Here's how the part is built. I have some questions about the finished solid (model axes, mm). A direction names the side the tool comes from. Coordinates: 2 decimals unless noted, no trailing zeros. Order: outer loops, then holes, each group sorted by start corner. A loop starts at its lowest first (then second) coordinate and runs counter-clockwise, first axis right, second up. Notation, with made-up numbers: M 6,55 L 24,55 A32 ccw 24,87 Z; hole C -40,35 d2. An arc over 180 degrees is marked long. Answer as CSV lines item,"result". Start each with the question number.
```python
from build123d import *

# Parameters (mm, degrees)
SKETCH1_R           = 15
BOSS_EXTRUDE1_DEPTH = 5
SKETCH2_R           = 5
BOSS_EXTRUDE2_DEPTH = 90
CUT_EXTRUDE1_START  = -15
CUT_EXTRUDE1_DEPTH  = 15
SKETCH4_W           = 2
SKETCH4_H           = 5.2
CUT_EXTRUDE2_DEPTH  = 99.17076958
FILLET1_R           = 10
FILLET2_R           = 2
CUT_EXTRUDE3_DEPTH  = 1
SKETCH6_R           = 13.5
SKETCH6_R_2         = 11.5
CUT_EXTRUDE4_DEPTH  = 1


with BuildPart() as part:
    # Sketch1 → Boss-Extrude1 (new body)
    with BuildSketch(Plane(origin=(0, 0, 0), x_dir=(1, 0, 0), z_dir=(0, 1, 0))):
        with Locations(Location((0, 0, 0), (0, 0, 270))):
            Circle(SKETCH1_R)
    extrude(amount=BOSS_EXTRUDE1_DEPTH)

    # Sketch2 → Boss-Extrude2 (add)
    with BuildSketch(Plane(origin=(0, 5, 0), x_dir=(1, 0, 0), z_dir=(0, 1, 0))):
        with Locations(Location((0, 0, 0), (0, 0, 90))):
            Circle(SKETCH2_R)
    extrude(amount=BOSS_EXTRUDE2_DEPTH)

    # Sketch3 → Cut-Extrude1 (cut)
    with BuildSketch(Plane(origin=(0, 95, 0), x_dir=(1, 0, 0), z_dir=(0, 1, 0)).offset(CUT_EXTRUDE1_START)):
        with BuildLine():
            Line((0, 5), (5, 0))
            ThreePointArc((5, 0), (3.535533906, 3.535533906), (0, 5))
        make_face()
    extrude(amount=CUT_EXTRUDE1_DEPTH, mode=Mode.SUBTRACT)

    # Sketch4 → Cut-Extrude2 (cut, through all)
    with BuildSketch(Plane(origin=(2.5, 0, -2.5), x_dir=(-0.7071067811865475, 0, -0.7071067811865477), z_dir=(0.7071067811865477, 0, -0.7071067811865475))):
        with Locations((0, 87.5)):
            Rectangle(SKETCH4_W, SKETCH4_H)
    extrude(amount=-CUT_EXTRUDE2_DEPTH, mode=Mode.SUBTRACT)

    # Fillet1
    fillet1_edges = [part.edges().sort_by_distance(p)[0] for p in [
        (0, 5, 5),
    ]]
    fillet(fillet1_edges, radius=FILLET1_R - 0.0001)  # a hair under: the kernel refuses the full size

    # Fillet2
    fillet2_edges = [part.edges().sort_by_distance(p)[0] for p in [
        (0, 5, -15),
    ]]
    fillet(fillet2_edges, radius=FILLET2_R)

    # Sketch5 → Cut-Extrude3 (cut)
    with BuildSketch(Plane.XZ):
        with BuildLine():
            Line((-0.690387564, 10.623320935), (9.77235282, 0.16058055))
            Line((9.77235282, 0.16058055), (7.687016282, -1.924755988))
            Line((7.687016282, -1.924755988), (-2.195796218, 3.006133435))
            add(Edge.make_bspline(
                [(-2.195796218, 3.006133435), (-2.307029511, 3.062113904), (-2.52269645, 3.170652781), (-2.833890677, 3.329506222), (-3.122930247, 3.477577181), (-3.391022331, 3.612480856), (-3.636978399, 3.737620248), (-3.85910859, 3.856159494), (-4.059958905, 3.960316417), (-4.186011343, 4.026707574), (-4.245075064, 4.057816127)],
                knots=[0, 0, 0, 0, 1.297460102, 2.515607, 3.640415016, 4.681187102, 5.642653462, 6.515599393, 7.304462283, 8, 8, 8, 8], degree=3))
            add(Edge.make_bspline(
                [(-4.245075064, 4.057816127), (-4.210973718, 3.991734504), (-4.138662994, 3.851610709), (-4.025441526, 3.629760807), (-3.897989309, 3.38652834), (-3.762956902, 3.118983989), (-3.620144132, 2.827316511), (-3.462218864, 2.515142559), (-3.297896109, 2.177641474), (-3.18347293, 1.945388515), (-3.124281795, 1.825244012)],
                knots=[0, 0, 0, 0, 0.714390188, 1.514839662, 2.392796159, 3.352429004, 4.393822708, 5.512665897, 6.71330155, 8, 8, 8, 8], degree=3))
            Line((-3.124281795, 1.825244012), (1.650357628, -7.961414642))
            Line((1.650357628, -7.961414642), (-0.212623141, -9.824395412))
            Line((-0.212623141, -9.824395412), (-10.675363526, 0.638344973))
            Line((-10.675363526, 0.638344973), (-9.34122891, 1.972479588))
            Line((-9.34122891, 1.972479588), (-0.585219295, -6.783530027))
            Line((-0.585219295, -6.783530027), (-6.300363526, 5.013344973))
            Line((-6.300363526, 5.013344973), (-5.050363526, 6.263344973))
            Line((-5.050363526, 6.263344973), (6.88172782, 0.382936319))
            Line((6.88172782, 0.382936319), (-2.02452218, 9.289186319))
            Line((-2.02452218, 9.289186319), (-0.690387564, 10.623320935))
        make_face()
    extrude(amount=-CUT_EXTRUDE3_DEPTH, mode=Mode.SUBTRACT)

    # Sketch6 → Cut-Extrude4 (cut)
    with BuildSketch(Plane.XZ):
        with Locations(Location((0, 0, 0), (0, 0, 270))):
            Circle(SKETCH6_R)
        with Locations(Location((0, 0, 0), (0, 0, 270))):
            Circle(SKETCH6_R_2, mode=Mode.SUBTRACT)
    extrude(amount=-CUT_EXTRUDE4_DEPTH, mode=Mode.SUBTRACT)


solid = part.part
```
1) If we mould it in two halves opening along Y, with no side actions, what happens to faces 1 (the face through (0, 0, 0)), 2 (the face through (0, 95, 0)), 3 (the face through (0, 84.9, 0)), 4 (the face through (0.832, 0.493, 3.364))? For each: released by +Y, released by -Y, zero draft, split by the parting line, or undercut.
2) Suppose I cut it at C-C on y = 8. Please give me the cut outline in (x, z), plus the area to 3 significant figures.
3) I need wall thicknesses on line 1 (X direction, y = 0.75, z = 0); line 2 (Z direction, x = 0, y = 26); line 3 (Y direction, x = -9.5, z = -3.5). Which ranges of each line are inside material? Lowest first, please. Write a range as [from, to].
4) Suppose I cut it at B-B on y = 44. Please give me the cut outline in (x, z), plus the area to 3 significant figures.
5) Which directions (+Z, -Z, +X, -X, +Y, -Y) give clear straight access to the entire face, cutting with the end or side of a thin tool? Please do faces 5 (the face through (-3.4, 0.49, -0.97)), 6 (the face through (-3, 54, 4)), 7 (the face through (3, 80, -3)), 8 (the face through (0, 90.1, 0)).
6) Suppose I cut it at A-A on y = 87.5. Please give me the cut outline in (x, z), plus the area to 3 significant figures.
7) Will these pins go through, and if not, where does the flat tip stop? pin 1 Ø5 at (x, z) = (9, -8.5) entering from +Y; pin 2 Ø1 at (x, z) = (-10.5, -12) entering from -Y; pin 3 Ø2 at (x, y) = (-5.5, 12.5) entering from +Z; pin 4 Ø5 at (x, y) = (-1.5, 81.5) entering from -Z.
Output:
1,face 1,"released by -Y"
1,face 2,"released by +Y"
1,face 3,"undercut"
1,face 4,"zero draft"
2,outline,"C 0,0 d15.72"
2,area,"194 mm²"
3,line 1,"[-15, -13.5], [-11.5, -10.04], [-7.37, -3.87], [-2.23, 3.83], [9.61, 11.5], [13.5, 15]"
3,line 2,"[-5, 5]"
3,line 3,"[0, 6.27]"
4,outline,"C 0,0 d10"
4,area,"78.5 mm²"
5,face 5,"-Y"
5,face 6,"+Y"
5,face 7,"-Z, +X, +Y"
5,face 8,"none"
6,outline,"M -4.17,2.76 A5 ccw 0,-5 L 1.79,-3.21 Z; M -2.76,4.17 L 3.21,-1.79 L 5,0 A5 ccw Z"
6,area,"54.4 mm²"
7,pin 1,"y = 6.41"
7,pin 2,"through"
7,pin 3,"z = 2.92"
7,pin 4,"z = -5"
